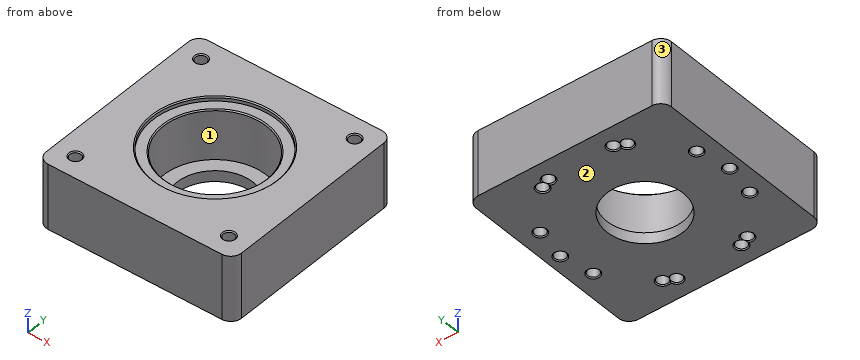
```python
from build123d import *

# Parameters (mm, degrees)
SKETCH1_R                         = 35
BOSS_EXTRUDE1_DEPTH               = 60
M12X1_75_TAPPED_HOLE1_D           = 10.2
M12X1_75_TAPPED_HOLE1_DEPTH       = 35.25
M12X1_75_TAPPED_HOLE1_CSINK_D     = 12.05
M12X1_75_TAPPED_HOLE1_CSINK_ANGLE = 90
M12X1_75_TAPPED_HOLE1_TIP         = 3.064389157
SKETCH5_R                         = 57.15
CUT_EXTRUDE1_DEPTH                = 4
CIRPATTERN1_COUNT                 = 6
SKETCH9_R                         = 47.5
CUT_EXTRUDE2_DEPTH                = 50
CHAMFER1_SIZE                     = 1
M12_TAPPED_HOLE2_D                = 10.2
M12_TAPPED_HOLE2_DEPTH            = 35.25
M12_TAPPED_HOLE2_CSINK_D          = 12.05
M12_TAPPED_HOLE2_CSINK_ANGLE      = 90
M12_TAPPED_HOLE2_TIP              = 3.064389157


with BuildPart() as part:
    # Sketch1 → Boss-Extrude1 (new body)
    with BuildSketch(Plane.XY):
        with BuildLine():
            Line((-80, -90), (80, -90))
            ThreePointArc((80, -90), (87.071067812, -87.071067812), (90, -80))
            Line((90, -80), (90, 80))
            ThreePointArc((90, 80), (87.071067812, 87.071067812), (80, 90))
            Line((80, 90), (-80, 90))
            ThreePointArc((-80, 90), (-87.071067812, 87.071067812), (-90, 80))
            Line((-90, 80), (-90, -80))
            ThreePointArc((-90, -80), (-87.071067812, -87.071067812), (-80, -90))
        make_face()
        Circle(SKETCH1_R, mode=Mode.SUBTRACT)
    extrude(amount=BOSS_EXTRUDE1_DEPTH)

    # M12x1.75 Tapped Hole1
    with Locations(Plane.XY.offset(60)):
        with Locations((-70.710678119, 70.710678119), (70.710678119, 70.710678119), (70.710678119, -70.710678119), (-70.710678119, -70.710678119)):
            CounterSinkHole(M12X1_75_TAPPED_HOLE1_D / 2, M12X1_75_TAPPED_HOLE1_CSINK_D / 2, depth=M12X1_75_TAPPED_HOLE1_DEPTH, counter_sink_angle=M12X1_75_TAPPED_HOLE1_CSINK_ANGLE)
            with Locations((0, 0, -(M12X1_75_TAPPED_HOLE1_DEPTH + M12X1_75_TAPPED_HOLE1_TIP / 2))):  # 118° drill point
                Cone(0, M12X1_75_TAPPED_HOLE1_D / 2, M12X1_75_TAPPED_HOLE1_TIP, mode=Mode.SUBTRACT)

    # Sketch5 → Cut-Extrude1 (cut)
    with BuildSketch(Plane.XY.offset(60)):
        Circle(SKETCH5_R)
    extrude(amount=-CUT_EXTRUDE1_DEPTH, mode=Mode.SUBTRACT)

    # Sketch8 → M12 Tapped Hole1 (revolve, cut)
    with BuildSketch(Plane(origin=(39, 67.549981495, 0), x_dir=(0, 1, 0), z_dir=(1, 0, 0))):
        Polygon((0, 0), (0, 38.314389157), (5.1, 35.25), (5.1, 0.925), (6.025, 0), align=None)
    m12_tapped_hole1 = revolve(axis=Axis((39, 67.549981495, -6.35), (0, 0, 1)), mode=Mode.SUBTRACT)

    # CirPattern1: M12 Tapped Hole1 ×6 about axis
    cirpattern1_axis = Axis((0, 0, 0), (0, 0, 1))
    for i in range(1, CIRPATTERN1_COUNT):
        add(m12_tapped_hole1.rotate(cirpattern1_axis, i * 360 / CIRPATTERN1_COUNT), mode=Mode.SUBTRACT)

    # Sketch9 → Cut-Extrude2 (cut)
    with BuildSketch(Plane.XY.offset(60)):
        Circle(SKETCH9_R)
    extrude(amount=-CUT_EXTRUDE2_DEPTH, mode=Mode.SUBTRACT)

    # Chamfer1
    chamfer1_edges = [part.edges().sort_by_distance(p)[0] for p in [
        (-57.15, 0, 60),
        (-47.5, 0, 56),
    ]]
    chamfer(chamfer1_edges, length=CHAMFER1_SIZE)

    # M12 Tapped Hole2
    with Locations(Plane(origin=(29.849307724, 72.062603536, 0), x_dir=(-1, 0, 0), z_dir=(0, 0, -1))):
        with Locations((0, 0), (59.698615448, 0), (101.91191126, -42.213295812), (101.91191126, -101.91191126), (59.698615448, -144.125207072), (0, -144.125207072), (-42.213295812, -101.91191126), (-42.213295812, -42.213295812)):
            CounterSinkHole(M12_TAPPED_HOLE2_D / 2, M12_TAPPED_HOLE2_CSINK_D / 2, depth=M12_TAPPED_HOLE2_DEPTH, counter_sink_angle=M12_TAPPED_HOLE2_CSINK_ANGLE)
            with Locations((0, 0, -(M12_TAPPED_HOLE2_DEPTH + M12_TAPPED_HOLE2_TIP / 2))):  # 118° drill point
                Cone(0, M12_TAPPED_HOLE2_D / 2, M12_TAPPED_HOLE2_TIP, mode=Mode.SUBTRACT)


solid = part.part
```
Work out the finished part from the listing and answer in its coordinate system (mm). Face numbers are marked on the shaded views. Give positions to 0.01 mm unless a question says otherwise; leave off trailing zeros. Loops run counter-clockwise (first coordinate to the right, second up) from the corner with the lowest first, then second, coordinate; pieces in that order, holes last. Notation, with made-up numbers: (45.5, 86.25) -> (90.5, 86.25) arc R15 ccw to (90.5, 90.25) -> close; hole circle Ø11 at (31.25, -4). An arc over 180 degrees is marked (long way). Put each result on its own line as item: value. Start each with the question number.
Item 1: The part is cut by section A-A (x = 0). Give the vertices of the cut face in (y, z).
Item 2: Each of these flat-tipped pins is pushed along its axis until it touches: P1, Ø11.5, axis at x = 70.71, y = -70.71, coming from the +Z side; P2, Ø6, axis at x = 70.71, y = 70.71, coming from the +Z side; P3, Ø9, axis at x = -29.85, y = -72.06, coming from the -Z side; P4, Ø16.5, axis at x = -78, y = 0, coming from the -Z side. Where does it stop, or does it pass through?
Item 3: Find the intervals of material crossed by L1, parallel to X at y = 0, z = 8; L2, parallel to X at y = -70.5, z = 47.5; L3, parallel to Y at x = -68.5, z = 22, in increasing order. Write a range as [from, to].
Item 4: The part is cut by section D-D (z = 44). Give the vertices of the cut face in (x, y), then the cut area to 3 significant figures.
Item 5: The part is cut by section B-B (z = 13.5). State how many separate pieces and enclosed holes the cut face has, then the cut area to 3 significant figures.
Item 6: The mould has two halves that part along Y. Classify the marked faces 1, 2 and 3: released by +Y, released by -Y, zero draft, split by the parting line, or undercut.
Answers below:
1. outline: (-90, 0) -> (-35, 0) -> (-35, 10) -> (-47.5, 10) -> (-47.5, 55) -> (-48.5, 56) -> (-57.15, 56) -> (-57.15, 59) -> (-58.15, 60) -> (-90, 60) -> close; (35, 0) -> (90, 0) -> (90, 60) -> (58.15, 60) -> (57.15, 59) -> (57.15, 56) -> (48.5, 56) -> (47.5, 55) -> (47.5, 10) -> (35, 10) -> close
2. P1: z = 59.73
2. P2: z = 23.49
2. P3: z = 35.61
2. P4: z = 0
3. L1: [-90, -83.1], [-72.9, -35], [35, 72.9], [83.1, 90]
3. L2: [-90, -75.81], [-65.62, 65.62], [75.81, 90]
3. L3: [-90, -33.5], [-26.2, 26.2], [33.5, 90]
4. outline: (-90, -80) arc R10 ccw to (-80, -90) -> (80, -90) arc R10 ccw to (90, -80) -> (90, 80) arc R10 ccw to (80, 90) -> (-80, 90) arc R10 ccw to (-90, 80) -> close; hole circle Ø10.2 at (-70.71, -70.71); hole circle Ø10.2 at (-70.71, 70.71); hole circle Ø95 at (0, 0); hole circle Ø10.2 at (70.71, -70.71); hole circle Ø10.2 at (70.71, 70.71)
4. area: 24,900 mm2
5. separate pieces: 1
5. enclosed holes: 15
5. area: 24,100 mm2
6. face 1: undercut
6. face 2: zero draft
6. face 3: released by +Y
